Source: three-view drawing plus pictorial views. Frame: mm from the lowest corner of the part. A direction names the side the tool comes from. Coordinates: 2 decimals unless noted, no trailing zeros. Order: outer loops, then holes, each group sorted by start corner. A loop starts at its lowest first (then second) coordinate and runs counter-clockwise, first axis right, second up. Notation, with made-up numbers: (-29, -0.5) - (13, -0.5) arc R26 cw to (13, 35.5) - close; hole circle Ø11 at (49.25, 54). An arc over 180 degrees is marked (long way). One line per question, with ' | ' between items.
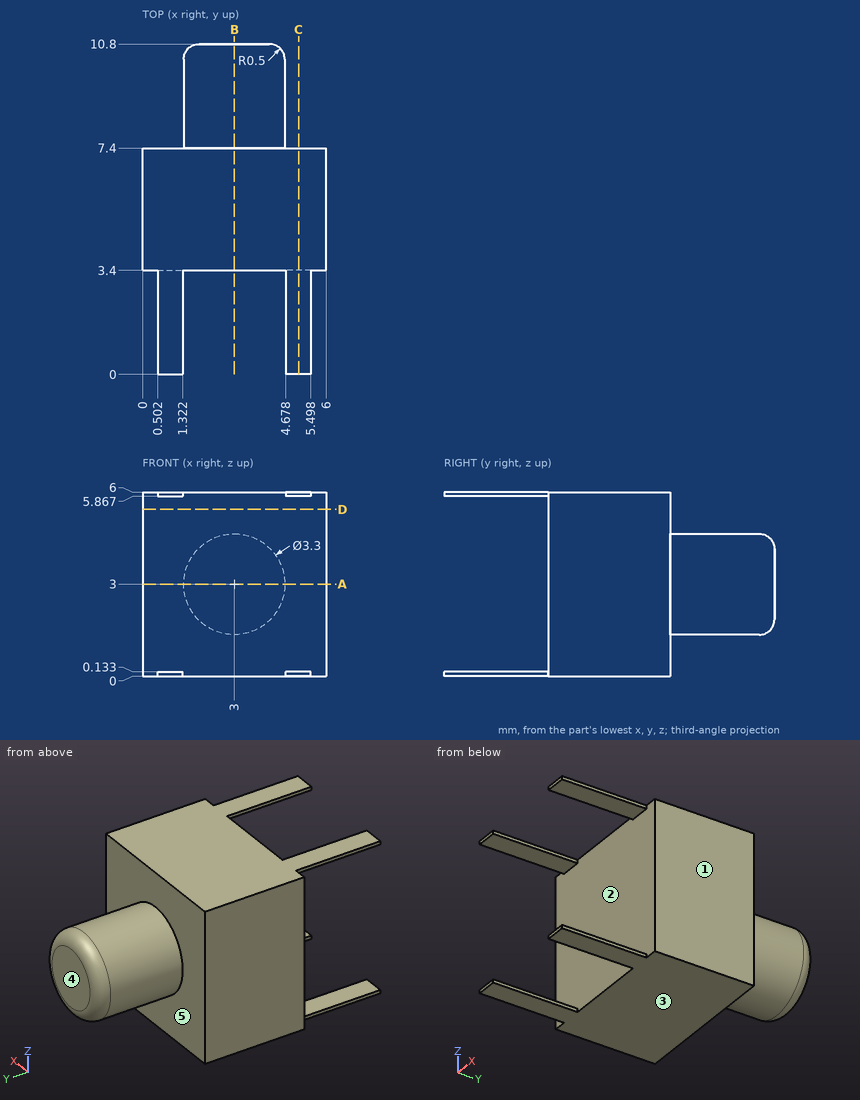
(1) Cut plane D-D (z = 5.45). Return the cut outline in (x, y), and give its area (3 significant figures).
Taken from the geometry:
outline: (0, 3.4) - (6, 3.4) - (6, 7.4) - (0, 7.4) - close | area: 24.0 mm²
(2) Set-up query: the marked faces 4 and 5. Return all of +Z, -Z, +X, -X, +Y, -Y with unobstructed straight access to the full face (end or side cutting, diameter ignored); none if empty.
Taken from the geometry:
face 4: +Z, -Z, +X, -X, +Y | face 5: +Y
(3) Cut plane A-A (z = 3). Return the cut outline in (x, y).
Taken from the geometry:
outline: (0, 3.4) - (6, 3.4) - (6, 7.4) - (4.65, 7.4) - (4.65, 10.3) arc R0.5 ccw to (4.15, 10.8) - (1.85, 10.8) arc R0.5 ccw to (1.35, 10.3) - (1.35, 7.4) - (0, 7.4) - close
(4) Cut plane C-C (x = 5.1). Return the cut outline in (y, z).
Taken from the geometry:
outline: (0, 0) - (7.4, 0) - (7.4, 6) - (0, 6) - (0, 5.87) - (3.4, 5.87) - (3.4, 0.13) - (0, 0.13) - close
(5) Cut plane B-B (x = 3). Return the cut outline in (y, z), and give its area (3 significant figures).
Taken from the geometry:
outline: (3.4, 0) - (7.4, 0) - (7.4, 1.35) - (10.3, 1.35) arc R0.5 ccw to (10.8, 1.85) - (10.8, 4.15) arc R0.5 ccw to (10.3, 4.65) - (7.4, 4.65) - (7.4, 6) - (3.4, 6) - close | area: 35.1 mm²
(6) Material intervals for L1, parallel to Y at x = 0.95, z = 3.6; L2, parallel to Y at x = 4.05, z = 2.9; L3, parallel to Z at x = 1.85, y = 8.75 (1 decimal), sorted ascending. Write a range as from..to.
Taken from the geometry:
L1: y = 3.4..7.4 | L2: y = 3.4..10.8 | L3: z = 1.8..4.2
(7) Pin query (flat end, axial travel): P1, Ø1.5, axis at x = 1, y = 9, coming from the -Z side; P2, Ø3, axis at x = 3, z = 3.5, coming from the -Y side. Return the tip coordinate at first contact, or that it passes through.
Taken from the geometry:
P1: stops at z = 1.92 | P2: stops at y = 3.4
(8) Pull-direction query (Z, two-part tool) for the marked faces 1, 2 and 3; classes: pulls with the +Z half, pulls with the -Z half, needs draft (parallel to the pull), parting line crosses it, or undercut.
Taken from the geometry:
face 1: needs draft | face 2: undercut | face 3: pulls with the -Z half
